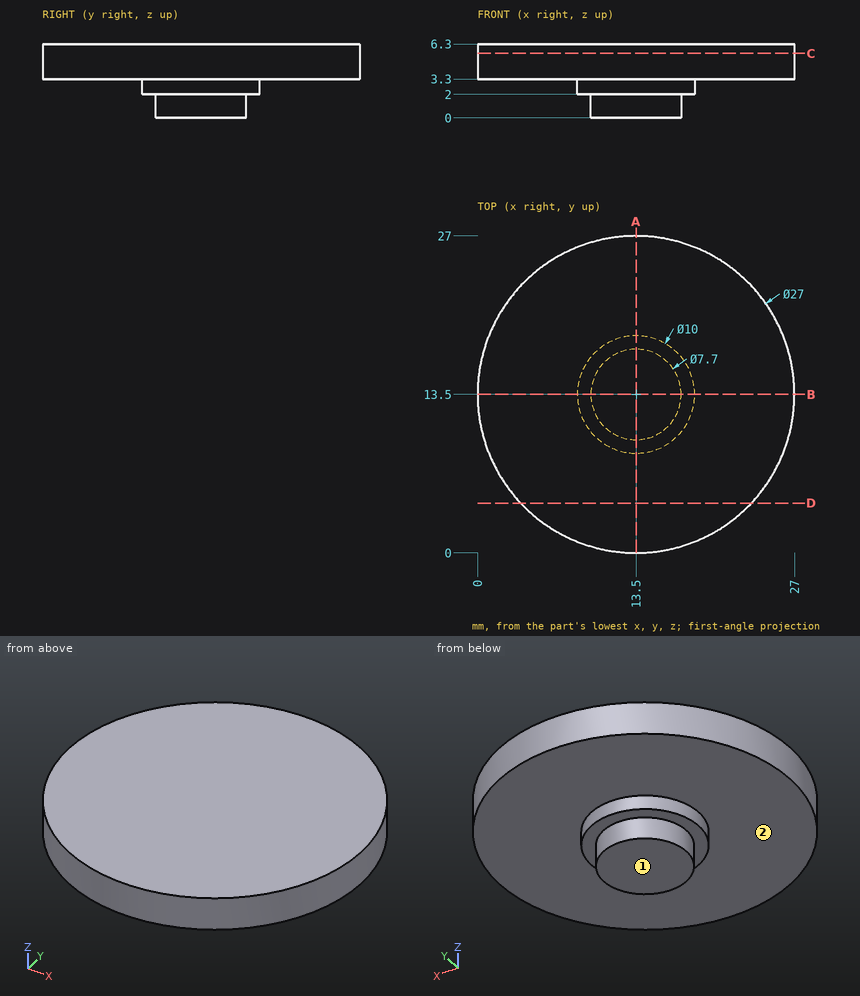
Geometry check sheet. Reference: drawing and pictorial views, mm from the part's lowest x, y, z. A direction names the side the tool comes from. Round coordinates to 2 decimals unless told otherwise and drop trailing zeros. Write each loop counter-clockwise with the first axis right and the second up, starting at its lowest first coordinate (ties: lowest second). Pieces come first, ordered by that corner, then holes. Notation, with made-up numbers: (14, 52.25) -> (48, 52.25) arc R9 ccw to (48, 57.25) -> close; hole circle Ø5 at (47.5, 24). An arc over 180 degrees is marked (long way). Put each result on its own line as item: value.
1) Cross-section at D-D, the plane y = 4.25. Enter the section's corners in (x, z), plus the area to 3 significant figures.
Recorded:
outline: (3.67, 3.3) -> (23.33, 3.3) -> (23.33, 6.3) -> (3.67, 6.3) -> close
area: 59.0 mm2
2) Thickness scan on probe 1 along Z at (x, y) = (10.5, 19); probe 2 along Y at (x, z) = (22.25, 3.5); probe 3 along X at (y, z) = (16, 2.5). Record the ranges inside material, lowest first. Write a range as from..to.
Recorded:
probe 1: z = 3.3..6.3
probe 2: y = 3.22..23.78
probe 3: x = 9.17..17.83
3) Cross-section at A-A, the plane x = 13.5. Enter the section's corners in (y, z).
Recorded:
outline: (0, 3.3) -> (8.5, 3.3) -> (8.5, 2) -> (9.65, 2) -> (9.65, 0) -> (17.35, 0) -> (17.35, 2) -> (18.5, 2) -> (18.5, 3.3) -> (27, 3.3) -> (27, 6.3) -> (0, 6.3) -> close
4) Cross-section at C-C, the plane z = 5.5. Enter the section's corners in (x, y).
Recorded:
outline: circle Ø27 at (13.5, 13.5)
5) Access from +Z, -Z, +X, -X, +Y, -Y to the whole of each face (thin tool, end or side, straight path). Record for the marked faces 1 and 2.
Recorded:
face 1: -Z, +X, -X, +Y, -Y
face 2: -Z
6) Depth check by flat-ended pin: P1, Ø1, axis at x = 9, z = 4.5, coming from the +Y side; P2, Ø6, axis at x = 11.5, y = 10.5, coming from the -Z side; P3, Ø1.5, axis at y = 12, z = 5, coming from the -X side; P4, Ø3, axis at y = 17, z = 2, coming from the +X side. Enter the tip coordinate at first touch or a pass-through.
Recorded:
P1: stops at y = 26.39
P2: stops at z = 0
P3: stops at x = 0.02
P4: stops at x = 26.72
